from build123d import *

# Parameters (mm, degrees)
SKETCH2_R            = 10.5
BOSS_EXTRUDE1_DEPTH  = 20
SKETCH3_R            = 12
CUT_EXTRUDE1_DEPTH   = 3
SKETCH4_OUTSIDE_W    = 47.968
SKETCH4_OUTSIDE_H    = 58.968
SKETCH4_OUTSIDE_R    = 19
CUT_EXTRUDE2_DEPTH   = 0.25
SKETCH5_OUTSIDE_W    = 47.968
SKETCH5_OUTSIDE_H    = 58.968
SKETCH5_OUTSIDE_R    = 19
CUT_EXTRUDE3_DEPTH   = 0.25
CUT_EXTRUDE4_START   = -1.5
CUT_EXTRUDE4_DEPTH   = 1.5
LPATTERN1_COUNT      = 6
LPATTERN1_PITCH      = 3
MIRROR3_START        = -1.5
MIRROR3_COPY_1_DEPTH = 1.5
MIRROR3_COPY_2_DEPTH = 1.5
MIRROR3_COPY_3_DEPTH = 1.5
MIRROR3_COPY_4_DEPTH = 1.5
MIRROR3_COPY_5_DEPTH = 1.5
SKETCH10_R           = 4
CUT_EXTRUDE5_DEPTH   = 9.5
SKETCH11_R           = 1.5
CUT_EXTRUDE6_DEPTH   = 4


with BuildPart() as part:
    # Sketch2 → Boss-Extrude1 (new body)
    with BuildSketch(Plane.XY):
        with BuildLine():
            Line((-17, 14.739402973), (-17, -14.739402973))
            ThreePointArc((-17, -14.739402973), (0, -22.5), (17, -14.739402973))
            Line((17, -14.739402973), (17, 14.739402973))
            ThreePointArc((17, 14.739402973), (0, 22.5), (-17, 14.739402973))
        make_face()
        Circle(SKETCH2_R, mode=Mode.SUBTRACT)
    extrude(amount=BOSS_EXTRUDE1_DEPTH)

    # Sketch3 → Cut-Extrude1 (cut)
    with BuildSketch(Plane(origin=(0, 0, 0), x_dir=(-1, 0, 0), z_dir=(0, 0, -1))):
        Circle(SKETCH3_R)
    extrude(amount=-CUT_EXTRUDE1_DEPTH, mode=Mode.SUBTRACT)

    # Sketch4 outside → Cut-Extrude2 (cut)
    with BuildSketch(Plane.XY.offset(20)):
        Rectangle(SKETCH4_OUTSIDE_W, SKETCH4_OUTSIDE_H)
        Circle(SKETCH4_OUTSIDE_R, mode=Mode.SUBTRACT)
    extrude(amount=-CUT_EXTRUDE2_DEPTH, mode=Mode.SUBTRACT)

    # Sketch5 outside → Cut-Extrude3 (cut)
    with BuildSketch(Plane(origin=(0, 0, 0), x_dir=(-1, 0, 0), z_dir=(0, 0, -1))):
        Rectangle(SKETCH5_OUTSIDE_W, SKETCH5_OUTSIDE_H)
        Circle(SKETCH5_OUTSIDE_R, mode=Mode.SUBTRACT)
    extrude(amount=-CUT_EXTRUDE3_DEPTH, mode=Mode.SUBTRACT)

    # Sketch8 → Cut-Extrude4 (cut)
    with BuildSketch(Plane.XY.offset(18.25).offset(CUT_EXTRUDE4_START)):
        with BuildLine():
            Line((17, 8.485281374), (17, 14.739402973))
            ThreePointArc((17, 14.739402973), (0, 22.5), (-17, 14.739402973))
            Line((-17, 14.739402973), (-17, 8.485281374))
            ThreePointArc((-17, 8.485281374), (0, 19), (17, 8.485281374))
        make_face()
    cut_extrude4 = extrude(amount=CUT_EXTRUDE4_DEPTH, mode=Mode.SUBTRACT)

    # LPattern1: Cut-Extrude4 ×6
    with Locations(*[(0, 0, -i * LPATTERN1_PITCH) for i in range(1, LPATTERN1_COUNT)]):
        add(cut_extrude4, mode=Mode.SUBTRACT)

    # Mirror3: Cut-Extrude4 across plane
    add(cut_extrude4.mirror(Plane.ZX), mode=Mode.SUBTRACT)

    # Mirror3 copy 1 sketch → Mirror3 copy 1 (cut)
    with BuildSketch(Plane.XY.offset(15.25).offset(MIRROR3_START)):
        with BuildLine():
            Line((17, -8.485281374), (17, -14.739402973))
            ThreePointArc((17, -14.739402973), (0, -22.5), (-17, -14.739402973))
            Line((-17, -14.739402973), (-17, -8.485281374))
            ThreePointArc((-17, -8.485281374), (0, -19), (17, -8.485281374))
        make_face()
    extrude(amount=MIRROR3_COPY_1_DEPTH, mode=Mode.SUBTRACT)

    # Mirror3 copy 2 sketch → Mirror3 copy 2 (cut)
    with BuildSketch(Plane.XY.offset(12.25).offset(MIRROR3_START)):
        with BuildLine():
            Line((17, -8.485281374), (17, -14.739402973))
            ThreePointArc((17, -14.739402973), (0, -22.5), (-17, -14.739402973))
            Line((-17, -14.739402973), (-17, -8.485281374))
            ThreePointArc((-17, -8.485281374), (0, -19), (17, -8.485281374))
        make_face()
    extrude(amount=MIRROR3_COPY_2_DEPTH, mode=Mode.SUBTRACT)

    # Mirror3 copy 3 sketch → Mirror3 copy 3 (cut)
    with BuildSketch(Plane.XY.offset(9.25).offset(MIRROR3_START)):
        with BuildLine():
            Line((17, -8.485281374), (17, -14.739402973))
            ThreePointArc((17, -14.739402973), (0, -22.5), (-17, -14.739402973))
            Line((-17, -14.739402973), (-17, -8.485281374))
            ThreePointArc((-17, -8.485281374), (0, -19), (17, -8.485281374))
        make_face()
    extrude(amount=MIRROR3_COPY_3_DEPTH, mode=Mode.SUBTRACT)

    # Mirror3 copy 4 sketch → Mirror3 copy 4 (cut)
    with BuildSketch(Plane.XY.offset(6.25).offset(MIRROR3_START)):
        with BuildLine():
            Line((17, -8.485281374), (17, -14.739402973))
            ThreePointArc((17, -14.739402973), (0, -22.5), (-17, -14.739402973))
            Line((-17, -14.739402973), (-17, -8.485281374))
            ThreePointArc((-17, -8.485281374), (0, -19), (17, -8.485281374))
        make_face()
    extrude(amount=MIRROR3_COPY_4_DEPTH, mode=Mode.SUBTRACT)

    # Mirror3 copy 5 sketch → Mirror3 copy 5 (cut)
    with BuildSketch(Plane.XY.offset(3.25).offset(MIRROR3_START)):
        with BuildLine():
            Line((17, -8.485281374), (17, -14.739402973))
            ThreePointArc((17, -14.739402973), (0, -22.5), (-17, -14.739402973))
            Line((-17, -14.739402973), (-17, -8.485281374))
            ThreePointArc((-17, -8.485281374), (0, -19), (17, -8.485281374))
        make_face()
    extrude(amount=MIRROR3_COPY_5_DEPTH, mode=Mode.SUBTRACT)

    # Sketch10 → Cut-Extrude5 (cut)
    with BuildSketch(Plane.ZY.offset(17)):
        with Locations((10, 0)):
            Circle(SKETCH10_R)
    extrude(amount=-CUT_EXTRUDE5_DEPTH, mode=Mode.SUBTRACT)

    # Sketch11 → Cut-Extrude6 (cut)
    with BuildSketch(Plane.ZY.offset(17)):
        with Locations((5.050252532, 4.949747468)):
            Circle(SKETCH11_R)
        with Locations((5.050252532, -4.949747468)):
            Circle(SKETCH11_R)
        with Locations((14.949747468, -4.949747468)):
            Circle(SKETCH11_R)
        with Locations((14.949747468, 4.949747468)):
            Circle(SKETCH11_R)
    cut_extrude6 = extrude(amount=-CUT_EXTRUDE6_DEPTH, mode=Mode.SUBTRACT)

    # Sketch14 → Cut-Revolve1 (revolve, cut)
    with BuildSketch(Plane(origin=(0, 0, 10), x_dir=(-1, 0, 0), z_dir=(0, 0, -1)), mode=Mode.PRIVATE) as cut_revolve1_sk:
        Polygon((-17, 0), (-11.5, 0), (-14.5, -3), (-17, -3), align=None)
    revolve(cut_revolve1_sk.sketch.rotate(Axis((17, 0, 10), (-1, 0, 0)), 270), axis=Axis((17, 0, 10), (-1, 0, 0)), mode=Mode.SUBTRACT)

    # Mirror4: Cut-Extrude6 across plane
    add(cut_extrude6.mirror(Plane(origin=(0, 0, 0), x_dir=(0, 0, 1), z_dir=(1, 0, 0))), mode=Mode.SUBTRACT)


solid = part.part
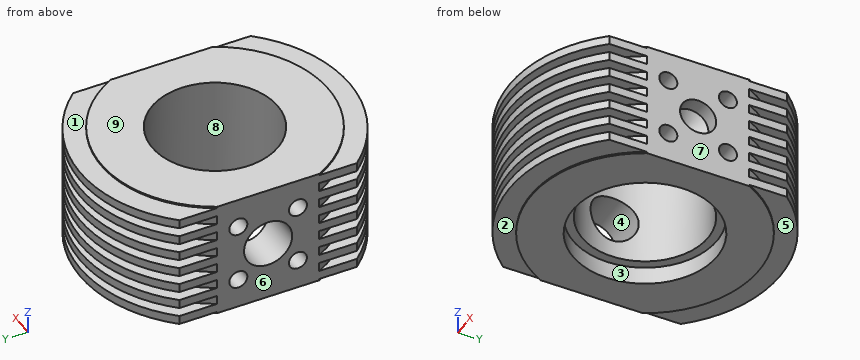
Geometry: final body of the model. Coordinates: model frame, mm. Face numbers are marked on the shaded views. A direction names the side the tool comes from. Round coordinates to 2 decimals unless told otherwise and drop trailing zeros. Loops run counter-clockwise (first coordinate to the right, second up) from the corner with the lowest first, then second, coordinate; pieces in that order, holes last. Notation, with made-up numbers: M -21.75,52.25 L 33.25,52.25 A13 ccw 33.25,57.25 Z; hole C 88,-27.75 d11. An arc over 180 degrees is marked long. One line per question, with ' | ' between items.
(1) Cut plane A-A on z = 2.25. Return the cut outline in (x, y), plus the area to 3 significant figures.
Check result:
outline: M -17,-8.49 A19 ccw 17,-8.49 L 17,8.49 A19 ccw -17,8.49 Z; hole C 0,0 d24 | area: 636 mm2
(2) Material intervals for line 1 along X through (y, z) = (-7.5, 6.75); line 2 along X through (y, z) = (5, 7.5); line 3 along Y through (x, z) = (-12, 17), sorted ascending. Write a range as from..to.
Check result:
line 1: x = -17..-7.35, 7.35..17 | line 2: x = -17..-9.23, 9.23..17 | line 3: y = -14.73..14.73
(3) Contact query for flat-ended pins moving along their axis: P1, Ø3.5, axis at y = -4.95, z = 5.05, coming from the +X side; P2, Ø1, axis at x = 12.5, z = 4, coming from the +Y side; P3, Ø0.9, axis at y = -5.5, z = 5.5, coming from the +X side. Output: stop coordinate, or through.
Check result:
P1: stops at x = 17 | P2: stops at y = 19.03 | P3: stops at x = 13
(4) Access query for the marked faces 1, 2, 3, 4 and 5. Directions: +Z, -Z, +X, -X, +Y, -Y. A direction counts if a zero-diameter tool reaches every point of the face in a straight line with its end or side. Return the directions, or none.
Check result:
face 1: +Z, +Y | face 2: -Z, -Y | face 3: -Z | face 4: -X | face 5: -Z, +Y
(5) Cut plane B-B on y = -1. Give the number of separate pieces and of enclosed holes in the cut face, plus the area to 3 significant figures.
Check result:
separate pieces: 3 | enclosed holes: 0 | area: 181 mm2
(6) Pull-direction query (X, two-part tool) for the marked faces 6, 7, 8 and 9; classes: +X half, -X half, draft (parallel to the pull), parting line (faces both ways), or undercut.
Check result:
face 6: -X half | face 7: +X half | face 8: undercut | face 9: draft
